Geometry: final body of the model. Coordinates: model frame, mm. Give positions to 0.01 mm unless a question says otherwise; leave off trailing zeros. Write each loop counter-clockwise with the first axis right and the second up, starting at its lowest first coordinate (ties: lowest second). Pieces come first, ordered by that corner, then holes. Notation, with made-up numbers: (26.25, -25.5) - (77.25, -25.5) arc R14 cw to (77.25, -15.5) - close; hole circle Ø6 at (63.5, 51.25). An arc over 180 degrees is marked (long way). One line per question, with ' | ' between items. Start each with the question number.
```python
from build123d import *

# Parameters (mm, degrees)
F0_W           = 22.225
F0_H           = 35.56
F1_DEPTH       = 1.5875
F3_D           = 2.9464
F3_CSINK_D     = 5.7404
F3_CSINK_ANGLE = 82


with BuildPart() as f1:
    # F0 (on Top) → F1 (new body)
    with BuildSketch(Plane.XY):
        Rectangle(F0_W, F0_H)
    extrude(amount=F1_DEPTH)

    # F3 (through all)
    with Locations(Plane.XY.offset(1.5875)):
        with Locations((0, 12.3825), (0, -12.3825)):
            CounterSinkHole(F3_D / 2, F3_CSINK_D / 2, counter_sink_angle=F3_CSINK_ANGLE)


solid = f1.part
```
1) Section B-B, the plane z = 0.85. Output: boundary loops of the cut face in (x, y).
2) Pull-direction query (Y, two-part tool) for faces 1 (the flat face through (11.112, 0, 1)), 2 (the flat face through (0, -17.78, 1)), 3 (the flat face through (0, 17.78, 1)); classes: +Y half, -Y half, draft (parallel to the pull), parting line (faces both ways), or undercut.
3) Line query: L1, parallel to Y at x = 1.75, z = 0.6; L2, parallel to Y at x = -1, z = 1.4; L3, parallel to X at y = 13, z = 0.4. Output: solid intervals per line, ascending.
4) Section A-A, the plane x = 0. Output: boundary loops of the cut face in (y, z), plus the area to 3 significant figures.
Answer key:
1) outline: (-11.11, -17.78) - (11.11, -17.78) - (11.11, 17.78) - (-11.11, 17.78) - close; hole circle Ø4.46 at (0, -12.38); hole circle Ø4.46 at (0, 12.38)
2) face 1: draft | face 2: -Y half | face 3: +Y half
3) L1: -17.78 to -13.37, -11.39 to 11.39, 13.37 to 17.78 | L2: -17.78 to -14.9, -9.87 to 9.87, 14.9 to 17.78 | L3: -11.11 to -1.73, 1.73 to 11.11
4) outline: (-17.78, 0) - (-13.87, 0) - (-15.25, 1.59) - (-17.78, 1.59) - close; (-10.89, 0) - (10.89, 0) - (9.51, 1.59) - (-9.51, 1.59) - close; (13.87, 0) - (17.78, 0) - (17.78, 1.59) - (15.25, 1.59) - close | area: 42.6 mm^2
